```python
from build123d import *

# Parameters (mm, degrees)
F1_DEPTH = 10
F4_D     = 6.6
F6_D     = 4.2
F6_DEPTH = 35
F6_TIP   = 1.2618073


with BuildPart() as f1:
    # F0 (on Right) → F1 (new body)
    with BuildSketch(Plane.YZ):
        Polygon((-0.5204892877, 337.3), (-90.8997518947, 0), (45.4005351965, 0), (45.4005351965, 337.3), (40.3610474387, 337.3), (22.4005351965, 319.3394877579), (4.4400229544, 337.3), align=None)
    extrude(amount=F1_DEPTH)

    # F4 (through all)
    with Locations(Plane(origin=(0, 0, 0), x_dir=(0, 1, 0), z_dir=(-1, 0, 0))):
        with Locations((10.4005351965, -240), (15.4005351965, -50), (-39.5994648035, -50)):
            Hole(F4_D / 2)

    # F6
    with Locations(Plane(origin=(0, 0, 0), x_dir=(1, 0, 0), z_dir=(0, 0, -1))):
        with Locations((5, 69.5994648035), (5, 19.5994648035), (5, -30.4005351965)):
            Hole(F6_D / 2, depth=F6_DEPTH)
            with Locations((0, 0, -(F6_DEPTH + F6_TIP / 2))):  # 118° drill point
                Cone(0, F6_D / 2, F6_TIP, mode=Mode.SUBTRACT)


solid = f1.part
```
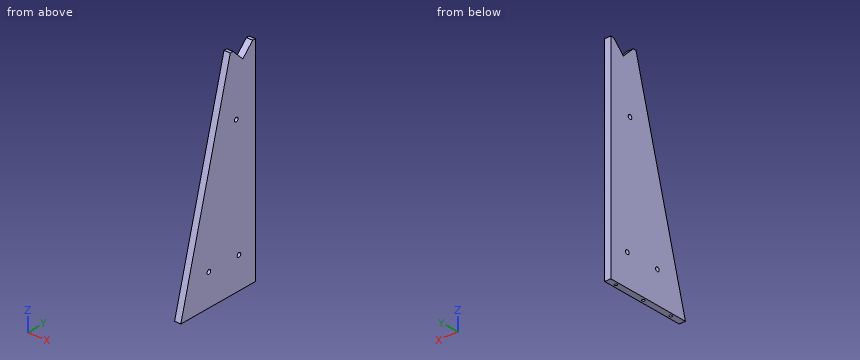
Verification items for the finished model (mm, model axes). Round coordinates to 2 decimals unless told otherwise and drop trailing zeros. Write each loop counter-clockwise with the first axis right and the second up, starting at its lowest first coordinate (ties: lowest second). Pieces come first, ordered by that corner, then holes. Notation, with made-up numbers: (-38, 85.25) - (20, 85.25) arc R14 cw to (20, 107.25) - close; hole circle Ø5 at (-5, -18). An arc over 180 degrees is marked (long way). Answer as a JSON object with one key per item and string values. Group by question number.
Q1. Section check A-A, the plane z = 240. Enter the section's corners in (x, y).
Q2. Section check B-B, the plane y = -77. Enter the section's corners in (x, z).
Q3. Section check C-C, the plane z = 69. Enter the section's corners in (x, y).
Q4. Go/stop test with flat-tipped pins: pin 1 Ø5 at (x, y) = (2, 7) entering from +Z; pin 2 Ø1 at (x, z) = (2.5, 38) entering from -Y; pin 3 Ø3.5 at (x, y) = (5, 30.4) entering from +Z; pin 4 Ø5.5 at (y, z) = (15.4, 50) entering from -X. Record where each tip stops, or that it passes through.
Q5. Thickness scan on line 1 (Y direction, x = 2.25, z = 50); line 2 (Y direction, x = 6, z = 48.5); line 3 (Y direction, x = 5, z = 21). Record the ranges inside material, lowest first.
Found:
{
 "1": {"outline": "(0, -26.59) - (10, -26.59) - (10, 7.1) - (0, 7.1) - close; (0, 13.7) - (10, 13.7) - (10, 45.4) - (0, 45.4) - close"},
 "2": {"outline": "(0, 0) - (10, 0) - (10, 51.87) - (0, 51.87) - close"},
 "3": {"outline": "(0, -72.41) - (10, -72.41) - (10, 45.4) - (0, 45.4) - close"},
 "4": {"pin 1": "stops at z = 337.24", "pin 2": "stops at y = -80.85", "pin 3": "stops at z = 329.09", "pin 4": "passes through"},
 "5": {"line 1": "y = -77.5 to -42.9, -36.3 to 12.1, 18.7 to 45.4", "line 2": "y = -77.9 to -42.54, -36.66 to 12.46, 18.34 to 45.4", "line 3": "y = -85.27 to -71.7, -67.5 to -21.7, -17.5 to 28.3, 32.5 to 45.4"}
}
